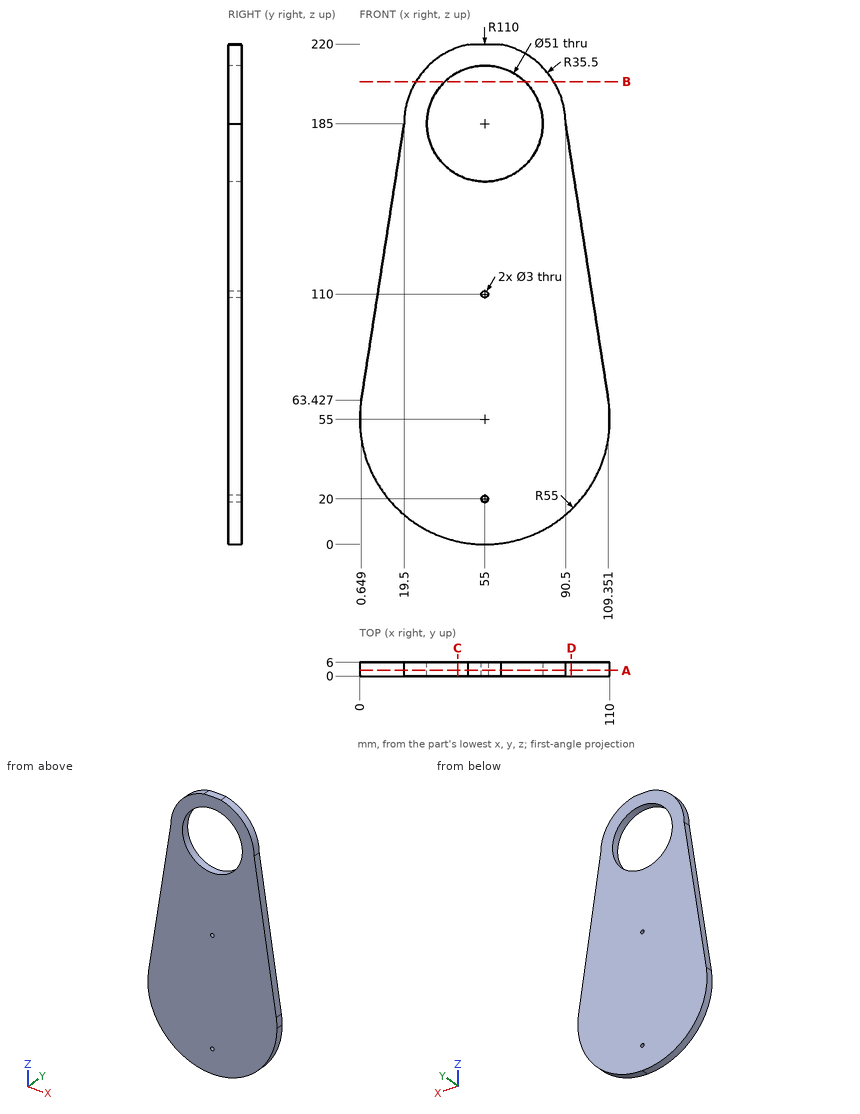
Can you work these out from the drawing? Everything is in mm from the part's minimum corner. Give positions to 0.01 mm unless a question says otherwise; leave off trailing zeros. Order: outer loops, then holes, each group sorted by start corner. A loop starts at its lowest first (then second) coordinate and runs counter-clockwise, first axis right, second up.
Item 1: If we section it at C-C, the plane x = 43: Write out the boundary of the cut face in (y, z) (1 decimal), plus the area to 3 significant figures.
Item 2: If we section it at B-B, the plane z = 203.5: Write out the boundary of the cut face in (x, y), plus the area to 3 significant figures.
Item 3: If we section it at A-A, the plane y = 2.5: Count the separate pieces of the cut face and the enclosed holes in it, plus the area to 3 significant figures.
Item 4: If we section it at D-D, the plane x = 93: Write out the boundary of the cut face in (y, z), plus the area to 3 significant figures.
Item 5: I need wall thicknesses on line 1 (Z direction, x = 55, y = 2.45); line 2 (X direction, y = 1.95, z = 185); line 3 (X direction, y = 4.15, z = 20) (1 decimal). Which ranges of each line are inside material? Lowest first, please.
Item 6: I'm going to push flat-ended pins straight in: pin 1 (3 mm diameter, centred on y = 3.5, z = 151.5, fed in from +X); pin 2 (2 mm diameter, centred on x = 63.5, y = 4.5, fed in from -Z). Where does each tip first touch, or does it pass through?
Values:
1. outline: (0, 1.3) - (6, 1.3) - (6, 162.5) - (0, 162.5) - close; (0, 207.5) - (6, 207.5) - (6, 218.4) - (0, 218.4) - close
1. area: 1,030 mm2
2. outline: (24.7, 0) - (37.45, 0) - (37.45, 6) - (24.7, 6) - close; (72.55, 0) - (85.3, 0) - (85.3, 6) - (72.55, 6) - close
2. area: 153 mm2
3. separate pieces: 1
3. enclosed holes: 3
3. area: 16,500 mm2
4. outline: (0, 15.24) - (6, 15.24) - (6, 168.88) - (0, 168.88) - close
4. area: 922 mm2
5. line 1: z = 0 to 18.5, 21.5 to 108.5, 111.5 to 159.5, 210.5 to 220
5. line 2: x = 19.5 to 29.5, 80.5 to 90.5
5. line 3: x = 12.6 to 53.5, 56.5 to 97.4
6. pin 1: stops at x = 95.93
6. pin 2: stops at z = 0.51
